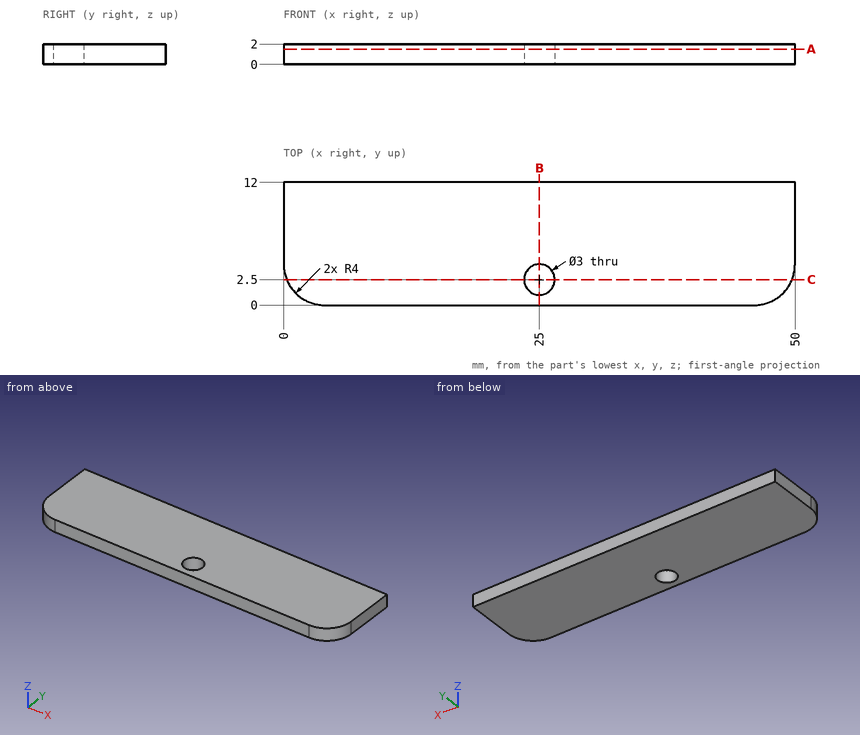
The drawing under review shows one solid part. Ordinate dimensions are in mm from its lowest x, y, z. Coordinates: 2 decimals unless noted, no trailing zeros. Write each loop counter-clockwise with the first axis right and the second up, starting at its lowest first coordinate (ties: lowest second). Pieces come first, ordered by that corner, then holes. Notation, with made-up numbers: (-4, 10.5) - (32, 10.5) arc R30 ccw to (32, 43.5) - close; hole circle Ø9 at (-27.5, 9). An arc over 180 degrees is marked (long way). Answer in a Markdown table with one row per item. Add a question column.
Q1. We need section C-C, the plane y = 2.5. State the section outline as (x, z) points, and give its area (3 significant figures).
Q2. For probe 1 along Y at (x, z) = (25, 1.55); probe 2 along X at (y, z) = (1.75, 1.7); probe 3 along Y at (x, z) = (3.5, 1.25), list the stretches that pass through material, from the lowest coordinate up.
Q3. We need section A-A, the plane z = 1.5. State the section outline as (x, y) points, and give its area (3 significant figures).
Q4. We need section B-B, the plane x = 25. State the section outline as (y, z) points.
Answer list:
| question | item | result |
|---|---|---|
| 1 | outline | (0.29, 0) - (23.5, 0) - (23.5, 2) - (0.29, 2) - close; (26.5, 0) - (49.71, 0) - (49.71, 2) - (26.5, 2) - close |
| 1 | area | 92.8 mm2 |
| 2 | probe 1 | y = 0 to 1, 4 to 12 |
| 2 | probe 2 | x = 0.69 to 23.7, 26.3 to 49.31 |
| 2 | probe 3 | y = 0.03 to 12 |
| 3 | outline | (0, 4) arc R4 ccw to (4, 0) - (46, 0) arc R4 ccw to (50, 4) - (50, 12) - (0, 12) - close; hole circle Ø3 at (25, 2.5) |
| 3 | area | 586 mm2 |
| 4 | outline | (0, 0) - (1, 0) - (1, 2) - (0, 2) - close; (4, 0) - (12, 0) - (12, 2) - (4, 2) - close |
